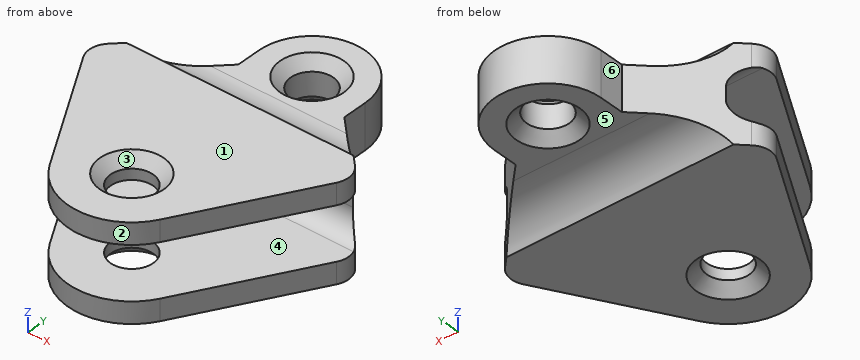
from build123d import *

# Parameters (mm, degrees)
SKETCH2_R           = 10
BOSS_EXTRUDE2_DEPTH = 22.5
CUT_EXTRUDE4_START  = -12
CUT_EXTRUDE4_DEPTH  = 12
FILLET7_R           = 25
CUT_EXTRUDE5_DEPTH  = 12.5
FILLET8_R           = 10
FILLET9_R           = 10
CHAMFER5_SIZE       = 5


with BuildPart() as part:
    # Sketch2 → Boss-Extrude2 (new body)
    with BuildSketch(Plane.XY):
        with BuildLine():
            Line((-25, 0), (-25, -11.491470389))
            Line((-25, -11.491470389), (-63.508529611, -50))
            Line((-63.508529611, -50), (-25.980762114, -115))
            ThreePointArc((-25.980762114, -115), (0, -130), (25.980762114, -115))
            Line((25.980762114, -115), (63.508529611, -50))
            Line((63.508529611, -50), (25, -11.491470389))
            Line((25, -11.491470389), (25, 0))
            ThreePointArc((25, 0), (0, 25), (-25, 0))
        make_face()
        with Locations(Location((0, 0, 0), (0, 0, 180))):
            Circle(SKETCH2_R, mode=Mode.SUBTRACT)
        with Locations(Location((0, -100, 0), (0, 0, 180))):
            Circle(SKETCH2_R, mode=Mode.SUBTRACT)
    extrude(amount=BOSS_EXTRUDE2_DEPTH)

    # Sketch7 → Cut-Extrude4 (cut)
    with BuildSketch(Plane.XY.offset(22.5).offset(CUT_EXTRUDE4_START)):
        with BuildLine():
            Line((-25, -11.491470389), (-53.508529611, -40))
            Line((-53.508529611, -40), (53.508529611, -40))
            Line((53.508529611, -40), (25, -11.491470389))
            Line((25, -11.491470389), (25, 0))
            ThreePointArc((25, 0), (0, 25), (-25, 0))
            Line((-25, 0), (-25, -11.491470389))
        make_face()
    extrude(amount=CUT_EXTRUDE4_DEPTH, mode=Mode.SUBTRACT)

    # Fillet7
    # the kernel refuses this fillet: 25 mm, written as the material it adds along each edge
    with BuildSketch(Plane(origin=(-106.893920871, -40, 10.5), x_dir=(0, 1, 0), z_dir=(1, 0, 0))) as fillet7_piece_1_section:
        with BuildLine():
            CenterArc((21.354156504, 25), FILLET7_R, 211.332251498, 58.667748502)
            Line((0, 12), (-0.42708313, 11.74))
            ThreePointArc((-0.42708313, 11.74), (-0.5, 6), (-0.5, 0))
            Line((-0.5, 0), (0, -0.5))
            Line((0, -0.5), (21.354156504, -0.5))
            Line((21.354156504, -0.5), (21.354156504, 0))
        make_face()
    fillet7_piece_1 = extrude(amount=213.787841742, mode=Mode.PRIVATE)
    fillet7_piece_1 = split(fillet7_piece_1, bisect_by=Plane(origin=(-24.314247143, -10.805717532, 13.775046533), z_dir=(0.7071067811865464, -0.7071067811865488, 0)), keep=Keep.TOP, mode=Mode.PRIVATE)
    fillet7_piece_1 = split(fillet7_piece_1, bisect_by=Plane(origin=(24.314247143, -10.805717532, 13.775046533), z_dir=(-0.7071067811865461, -0.7071067811865489, 0)), keep=Keep.TOP, mode=Mode.PRIVATE)
    add(fillet7_piece_1)

    # Sketch8 → Cut-Extrude5 (cut)
    with BuildSketch(Plane(origin=(0, 0, 0), x_dir=(-1, 0, 0), z_dir=(0, 0, -1))):
        with BuildLine():
            Line((-51.508529611, -38), (51.508529611, -38))
            Line((51.508529611, -38), (63.508529611, -50))
            Line((63.508529611, -50), (25.980762114, -115))
            ThreePointArc((25.980762114, -115), (0, -130), (-25.980762114, -115))
            Line((-25.980762114, -115), (-63.508529611, -50))
            Line((-63.508529611, -50), (-51.508529611, -38))
        make_face()
    extrude(amount=-CUT_EXTRUDE5_DEPTH, mode=Mode.SUBTRACT)

    # Fillet8
    fillet8_edges = [part.edges().sort_by_distance(p)[0] for p in [
        (0, -38, 12.5),
    ]]
    fillet(fillet8_edges, radius=FILLET8_R)

    # Fillet9
    fillet9_edges = [part.edges().sort_by_distance(p)[0] for p in [
        (-63.508529611, -50, 17.5),
        (63.508529611, -50, 17.5),
    ]]
    fillet(fillet9_edges, radius=FILLET9_R)

    # Chamfer5
    chamfer5_edges = [part.edges().sort_by_distance(p)[0] for p in [
        (10, -100, 22.5),
        (10, 0, 10.5),
    ]]
    chamfer(chamfer5_edges, length=CHAMFER5_SIZE)

    # Mirror3: part across plane


with BuildPart() as part_1:
    add(part.part)
    add(part.part.mirror(Plane(origin=(0, -100, 0), x_dir=(1, 0, 0), z_dir=(0, 0, 1))))


solid = part_1.part
Geometry check sheet. Reference: the model listing, model coordinates, mm. Face numbers are marked on the shaded views. A direction names the side the tool comes from. Round coordinates to 2 decimals unless told otherwise and drop trailing zeros. Write each loop counter-clockwise with the first axis right and the second up, starting at its lowest first coordinate (ties: lowest second). Pieces come first, ordered by that corner, then holes.
Item 1: Access from +Z, -Z, +X, -X, +Y, -Y to the whole of each face (thin tool, end or side, straight path). Record for the marked faces 4, 5 and 6.
Determined:
face 4: +X, -X, -Y
face 5: -Z, +X, -X, +Y
face 6: +Z, -Z, -X, +Y
Item 2: Section check B-B (y = -100). Record the boundary of the cut face in (x, z).
Determined:
outline: (-34.64, -22.5) - (-15, -22.5) - (-10, -17.5) - (-10, -12.5) - (-34.64, -12.5) - close; (-34.64, 12.5) - (-10, 12.5) - (-10, 17.5) - (-15, 22.5) - (-34.64, 22.5) - close; (10, -17.5) - (15, -22.5) - (34.64, -22.5) - (34.64, -12.5) - (10, -12.5) - close; (10, 12.5) - (34.64, 12.5) - (34.64, 22.5) - (15, 22.5) - (10, 17.5) - close
Item 3: Section check C-C (y = -61). Record the boundary of the cut face in (x, z), plus the area to 3 significant figures.
Determined:
outline: (-57.16, -22.5) - (57.16, -22.5) - (57.16, -12.5) - (-57.16, -12.5) - close; (-57.16, 12.5) - (57.16, 12.5) - (57.16, 22.5) - (-57.16, 22.5) - close
area: 2,290 mm2
Item 4: Material ranges on line 1 along Z through (x, y) = (15.5, -55); line 2 along Y through (x, z) = (0, 1.25); line 3 along X through (y, z) = (-100, -14), recorded low to high.
Determined:
line 1: z = -22.5 to -12.5, 12.5 to 22.5
line 2: y = -38 to -10, 10 to 25
line 3: x = -34.64 to -10, 10 to 34.64
Item 5: Mould release check, pull along X, two halves, no side actions. Record for the marked faces 1, 2 and 3: +X half, -X half, draft (parallel to the pull), parting line (faces both ways), or undercut.
Determined:
face 1: draft
face 2: parting line
face 3: undercut
Item 6: Section check D-D (x = 38). Record the boundary of the cut face in (y, z).
Determined:
outline: (-94.18, -22.5) - (-40, -22.5) arc R25 cw to (-24.49, -11.19) - (-24.49, 11.19) arc R25 cw to (-40, 22.5) - (-94.18, 22.5) - (-94.18, 12.5) - (-48, 12.5) arc R10 cw to (-38, 2.5) - (-38, -2.5) arc R10 cw to (-48, -12.5) - (-94.18, -12.5) - close
Item 7: Go/stop test with flat-tipped pins: pin 1 Ø4 at (x, z) = (5.5, -1) entering from -Y; pin 2 Ø3 at (y, z) = (-73.5, 16) entering from -X; pin 3 Ø12 at (x, z) = (-20, -1.5) entering from +Y; pin 4 Ø8 at (x, z) = (1, -15.5) entering from -Y. Record where each tip stops, or that it passes through.
Determined:
pin 1: stops at y = -38.01
pin 2: stops at x = -50.81
pin 3: stops at y = 20.71
pin 4: stops at y = -130
Item 8: Section check A-A (x = 0). Give the number of separate pieces and of enclosed holes in the cut face, plus the area to 3 significant figures.
Determined:
separate pieces: 4
enclosed holes: 0
area: 2,390 mm2
